The listing builds one solid part. Answer for the finished solid, in the listing's coordinates (mm). A direction names the side the tool comes from. Give positions to 0.01 mm unless a question says otherwise; leave off trailing zeros. Write each loop counter-clockwise with the first axis right and the second up, starting at its lowest first coordinate (ties: lowest second). Pieces come first, ordered by that corner, then holes. Notation, with made-up numbers: M 37,46 L 90,46 A9 ccw 90,62 Z; hole C 10,18.25 d11. An arc over 180 degrees is marked long. Answer as a JSON object with one key per item and string values.
```python
from build123d import *

# Parameters (mm, degrees)
SKETCH1_W               = 1143
SKETCH1_H               = 457.2
TABLETOP_DEPTH          = 50.8
PROFILE_R               = 24.13
MIRROR2_COPY_1_SKETCH_R = 24.13


with BuildPart() as part:
    # Sketch1 → TableTop (new body)
    with BuildSketch(Plane.XY):
        with Locations((571.5, 228.6)):
            Rectangle(SKETCH1_W, SKETCH1_H)
    extrude(amount=TABLETOP_DEPTH)

    # Sweep1: sweep along a path in Sketch11
    with BuildLine(Plane(origin=(0, 381, 0), x_dir=(1, 0, 0), z_dir=(0, 1, 0))) as sweep1_path:
        Line((76.2, -50.8), (50.297706266, -177.8))
        ThreePointArc((50.297706266, -177.8), (10.572817848, -428.926986426), (-6.770877712, -682.584287318))
    # Profile → Sweep1 (sweep)
    with BuildSketch(Plane.XY.offset(50.8)):
        with Locations((76.2, 381)):
            Circle(PROFILE_R)
    sweep1 = sweep(path=sweep1_path.line)

    # Mirror1: Sweep1 across plane
    add(sweep1.mirror(Plane(origin=(571.5, 0, 0), x_dir=(0, 0, 1), z_dir=(1, 0, 0))))

    # Mirror2: Sweep1 across plane
    add(sweep1.mirror(Plane.ZX.offset(228.6)))

    # Mirror2 copy 1: sweep along a path in Mirror2 copy 1 path
    with BuildLine(Plane(origin=(1143, 76.2, 0), x_dir=(-1, 0, 0), z_dir=(0, -1, 0))) as mirror2_copy_1_path:
        Line((76.2, -50.8), (50.297706266, -177.8))
        ThreePointArc((50.297706266, -177.8), (10.572817848, -428.926986426), (-6.770877712, -682.584287318))
    # Mirror2 copy 1 sketch → Mirror2 copy 1 (sweep)
    with BuildSketch(Plane(origin=(1143, 457.2, 50.8), x_dir=(-1, 0, 0), z_dir=(0, 0, 1))):
        with Locations((76.2, 381)):
            Circle(MIRROR2_COPY_1_SKETCH_R)
    sweep(path=mirror2_copy_1_path.line)


solid = part.part
```
1. The mould has two halves that part along X. Classify faces 4 (the flat face through (1143, 225, 25)), 5 (the flat face through (563, 232, 0)), 6 (the flat face through (-7.103, 381.338, 682.644)): released by +X, released by -X, zero draft, split by the parting line, or undercut.
Verdict:
{"face 4": "released by +X", "face 5": "zero draft", "face 6": "undercut"}
2. A cutting plane is placed at B-B, the plane x = 791.5. Give the vertices of the cut face in (y, z).
Verdict:
{"outline": "M 0,0 L 457.2,0 L 457.2,50.8 L 0,50.8 Z"}
3. For faces 1 (the flat face through (-7.103, 75.862, 682.644)), 2 (the flat face through (0, 225, 25)), 3 (the flat face through (563, 457.2, 25)), determine the directions among +Z, -Z, +X, -X, +Y, -Y from which every point of the face is accessible in a straight line to the end or side of a thin tool.
Verdict:
{"face 1": "+Z, +Y, -Y", "face 2": "-Z, -X, +Y, -Y", "face 3": "+Z, -Z, +X, -X, +Y"}
4. A cutting plane is placed at A-A, the plane y = 246. Give the vertices of the cut face in (x, z), plus the area to 3 significant figures.
Verdict:
{"outline": "M 0,0 L 1143,0 L 1143,50.8 L 0,50.8 Z", "area": "58,100 mm2"}
5. Consider line 1 along Z through (x, y) = (27, 258); line 2 along X through (y, z) = (64, 185.5); line 3 along X through (y, z) = (95, 564). Determine where each line is inside the solid, lowest interval first.
Verdict:
{"line 1": "z = 0 to 50.8", "line 2": "x = 27.93 to 69.55, 1073.45 to 1115.07", "line 3": "x = -16.33 to 13.38, 1129.62 to 1159.33"}
6. A flat-ended cylindrical pin translates along its axis: pin 1 (4 mm diameter, centred on x = 999, y = 207, fed in from +Z). Find the tip coordinate at first contact, or state that the pin passes through.
Verdict:
{"pin 1": "stops at z = 50.8"}
7. A cutting plane is placed at C-C, the plane z = 207. Count the separate pieces of the cut face and the enclosed holes in it, plus the area to 3 significant figures.
Verdict:
{"separate pieces": "4", "enclosed holes": "0", "area": "7,300 mm2"}
